Verification items for the finished model (mm, model axes). A direction names the side the tool comes from. Give positions to 0.01 mm unless a question says otherwise; leave off trailing zeros. Write each loop counter-clockwise with the first axis right and the second up, starting at its lowest first coordinate (ties: lowest second). Pieces come first, ordered by that corner, then holes. Notation, with made-up numbers: (-17.5, -4.75) -> (-11.5, -4.75) arc R23 cw to (-11.5, 28.25) -> close; hole circle Ø4 at (51, 36.5). An arc over 180 degrees is marked (long way). Answer as CSV lines item,"result". Start each with the question number.
1) Sectioned sample at A-A on z = 0. Record the cut outline in (x, y), and give its area (3 significant figures).
2) Sectioned sample at C-C on x = -164. Record the cut outline in (y, z).
3) Mould release check, pull along X, two halves, no side actions. Record for faces 4 (the flat face through (-171.45, -5, 5)), 5 (the flat face through (-177.8, 12.4, -4)), 6 (the flat face through (215.9, 0, 0)): released by +X, released by -X, zero draft, split by the parting line, or undercut.
4) Gauge pin test, flat ends, axial feed: pin 1 Ø8 at (x, z) = (-40, -12) entering from +Y; pin 2 Ø6 at (x, z) = (-130, -4) entering from +Y; pin 3 Ø12 at (x, y) = (-44.5, 4) entering from -Z. Record the tip position at first contact, or that the pin passes through.
5) Material ranges on L1, parallel to X at y = -12, z = 4.5; L2, parallel to X at y = 5, z = 7; L3, parallel to Y at x = 94, z = 0, recorded low to high.
6) Tool access check on faces 1 (the cylindrical face through (-2.4, -6.2, 1.38)), 2 (the cylindrical face through (-196.583, 11.267, -5.86)), 3 (the cylindrical face through (197.12, -12.4, 2.75)). Record the directions out of +Z, -Z, +X, -X, +Y, -Y that give a thin tool (end or side, any length) a straight path to the whole face; none if there is none.
```python
from build123d import *

# Parameters (mm, degrees)
BOSS_EXTRUDE1_DEPTH      = 171.45
BOSS_EXTRUDE1_DEPTH_BACK = 171.45
SKETCH2_R                = 6.35
SKETCH3_R                = 19.05
BOSS_EXTRUDE2_DEPTH      = 6.35
BOSS_EXTRUDE4_START      = 6.35
SKETCH7_R                = 19.05
BOSS_EXTRUDE4_DEPTH      = 6.35
SKETCH9_R                = 12.7
BOSS_EXTRUDE6_DEPTH      = 38.1
BOSS_EXTRUDE7_START      = 38.1
SKETCH10_R               = 12.7
BOSS_EXTRUDE7_DEPTH      = 38.1


with BuildPart() as part:
    # Sketch2 → Boss-Extrude1 (new, two sides: drawn at the far end of the back side and taken through both)
    with BuildSketch(Plane(origin=(0, 0, 0), x_dir=(0, 0, -1), z_dir=(1, 0, 0)).offset(-BOSS_EXTRUDE1_DEPTH_BACK)):
        Circle(SKETCH2_R)
    extrude(amount=BOSS_EXTRUDE1_DEPTH + BOSS_EXTRUDE1_DEPTH_BACK)

    # Sketch3 → Boss-Extrude2 (add)
    with BuildSketch(Plane(origin=(171.45, 0, 0), x_dir=(0, 0, -1), z_dir=(1, 0, 0))):
        Circle(SKETCH3_R)
    extrude(amount=BOSS_EXTRUDE2_DEPTH)

    # Sketch7 → Boss-Extrude4 (add)
    with BuildSketch(Plane.ZY.offset(171.45).offset(BOSS_EXTRUDE4_START)):
        with Locations(Location((0, 0, 0), (0, 0, 180))):
            Circle(SKETCH7_R)
    extrude(amount=-BOSS_EXTRUDE4_DEPTH)

    # Sketch9 → Boss-Extrude6 (add)
    with BuildSketch(Plane.ZY.offset(177.8)):
        with Locations(Location((0, 0, 0), (0, 0, 180))):
            Circle(SKETCH9_R)
    extrude(amount=BOSS_EXTRUDE6_DEPTH)

    # Sketch10 → Boss-Extrude7 (add)
    with BuildSketch(Plane(origin=(177.8, 0, 0), x_dir=(0, 0, -1), z_dir=(1, 0, 0)).offset(BOSS_EXTRUDE7_START)):
        Circle(SKETCH10_R)
    extrude(amount=-BOSS_EXTRUDE7_DEPTH)


solid = part.part
```
Ans:
1,outline,"(-215.9, -12.7) -> (-177.8, -12.7) -> (-177.8, -19.05) -> (-171.45, -19.05) -> (-171.45, -6.35) -> (171.45, -6.35) -> (171.45, -19.05) -> (177.8, -19.05) -> (177.8, -12.7) -> (215.9, -12.7) -> (215.9, 12.7) -> (177.8, 12.7) -> (177.8, 19.05) -> (171.45, 19.05) -> (171.45, 6.35) -> (-171.45, 6.35) -> (-171.45, 19.05) -> (-177.8, 19.05) -> (-177.8, 12.7) -> (-215.9, 12.7) -> close"
1,area,"6,770 mm²"
2,outline,"circle Ø12.7 at (0, 0)"
3,face 4,"undercut"
3,face 5,"released by -X"
3,face 6,"released by +X"
4,pin 1,"passes through"
4,pin 2,"stops at y = 6.27"
4,pin 3,"stops at z = -6.35"
5,L1,"x = -177.8 to -171.45, 171.45 to 177.8"
5,L2,"x = -215.9 to -171.45, 171.45 to 215.9"
5,L3,"y = -6.35 to 6.35"
6,face 1,"none"
6,face 2,"-X"
6,face 3,"+X"
